Answer from the drawing. Dimensions are ordinates in mm from the lowest x, y and z of the part. A direction names the side the tool comes from. Give positions to 0.01 mm unless a question says otherwise; leave off trailing zeros. Order: outer loops, then holes, each group sorted by start corner. A loop starts at its lowest first (then second) coordinate and runs counter-clockwise, first axis right, second up. Notation, with made-up numbers: (69, -10.75) - (106, -10.75) arc R5 cw to (106, -3.75) - close; hole circle Ø4 at (72.5, 72.25). An arc over 180 degrees is marked (long way). Answer in a Markdown table with one row per item.
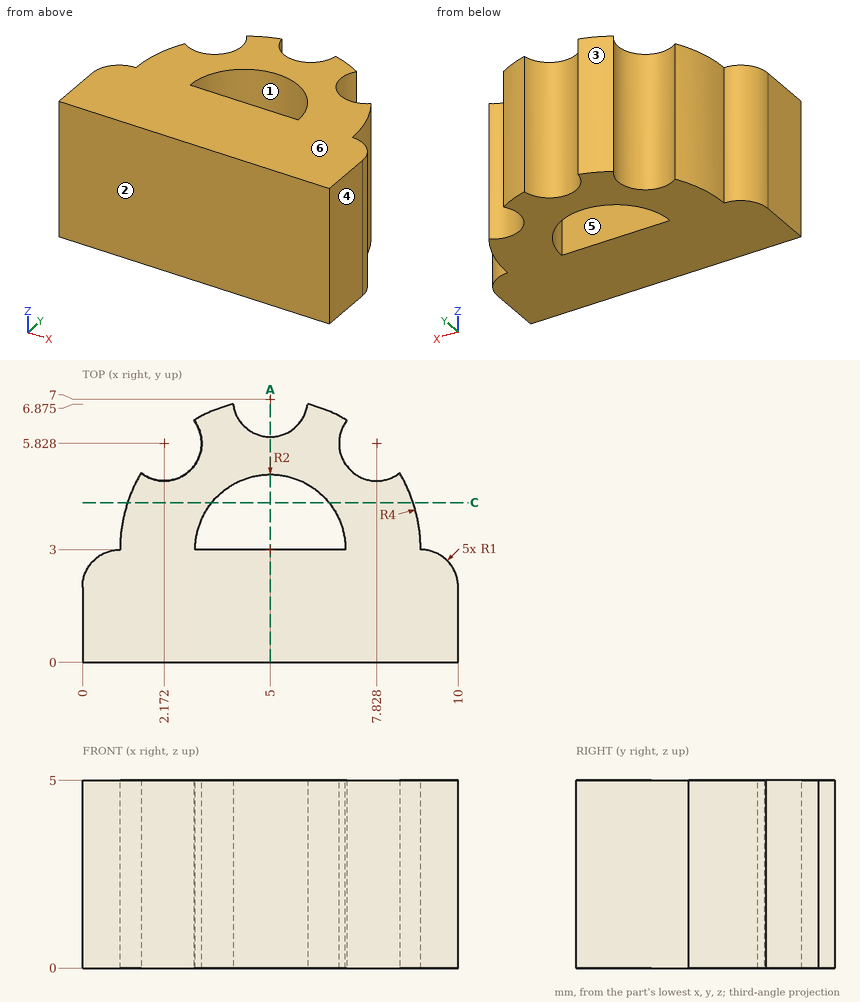
Item 1: Determine the mould class of the marked faces 1, 2, 3 and 4 for opening direction Y: pulls with the +Y half, pulls with the -Y half, needs draft (parallel to the pull), parting line crosses it, or undercut.
Answer block:
| item | result |
|---|---|
| face 1 | undercut |
| face 2 | pulls with the -Y half |
| face 3 | pulls with the +Y half |
| face 4 | needs draft |
Item 2: Consider line 1 (Y direction, x = 5, z = 0.65); line 2 (Y direction, x = 6.5, z = 4.75) (1 decimal); line 3 (X direction, y = 4, z = 3.35). Determine where each line is inside the solid, lowest interval first.
Answer block:
| item | result |
|---|---|
| line 1 | 0 to 3, 5 to 6 |
| line 2 | 0 to 3, 4.3 to 6.7 |
| line 3 | 1.13 to 3.27, 6.73 to 8.87 |
Item 3: This flat-tipped pin is pushed along its axis until it touches: P1, Ø1.2, axis at x = 5, z = 1.5, coming from the +Y side. Where does it stop, or does it pass through?
Answer block:
| item | result |
|---|---|
| P1 | y = 6.2 |
Item 4: Which of the six approach directions +Z, -Z, +X, -X, +Y, -Y give full straight-line access (tool end or side, diameter ignored) to the marked faces 5 and 6?
Answer block:
| item | result |
|---|---|
| face 5 | +Z, -Z |
| face 6 | +Z, +X, -X, +Y, -Y |
Item 5: Find section A-A on x = 5. Write down the section's boundary in (y, z).
Answer block:
| item | result |
|---|---|
| outline | (0, 0) - (3, 0) - (3, 5) - (0, 5) - close; (5, 0) - (6, 0) - (6, 5) - (5, 5) - close |
Item 6: Find section C-C on y = 4.25. Write down the section's boundary in (x, z).
Answer block:
| item | result |
|---|---|
| outline | (1.2, 0) - (3.44, 0) - (3.44, 5) - (1.2, 5) - close; (6.56, 0) - (8.8, 0) - (8.8, 5) - (6.56, 5) - close |
